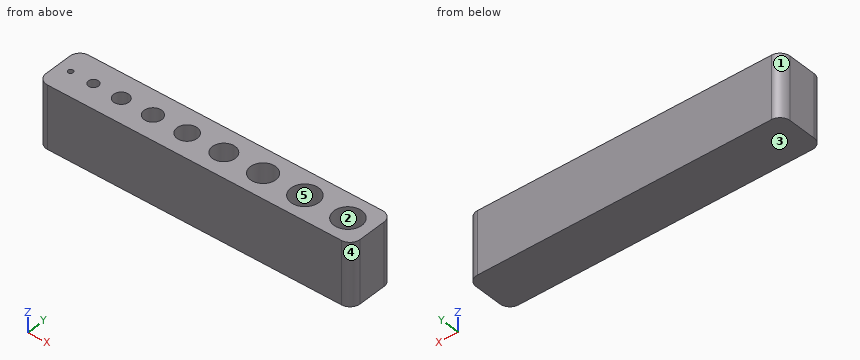
```python
from build123d import *

# Parameters (mm, degrees)
F0_W          = 62
F0_H          = 9.5
F0_R          = 0.5
F0_R_2        = 1
F0_R_3        = 1.5
F0_R_4        = 1.75
F0_R_5        = 2
F0_R_6        = 2.25
F0_R_7        = 2.5
F0_R_8        = 2.75
F1_DEPTH      = 12
F1_DEPTH_BACK = 0.4
F2_DEPTH      = 0.4
F3_R          = 2


with BuildPart() as f1:
    # F0 (on Top) → F1 (new body, two sides)
    with BuildSketch(Plane.XY) as f1_sk:
        with Locations((-1.75, 0)):
            Rectangle(F0_W, F0_H)
        with Locations((-30.25, 0)):
            Circle(F0_R, mode=Mode.SUBTRACT)
        with Locations((-25.75, 0)):
            Circle(F0_R_2, mode=Mode.SUBTRACT)
        with Locations((-20.25, 0)):
            Circle(F0_R_3, mode=Mode.SUBTRACT)
        with Locations((-14, 0)):
            Circle(F0_R_4, mode=Mode.SUBTRACT)
        with Locations((-7.25, 0)):
            Circle(F0_R_5, mode=Mode.SUBTRACT)
        Circle(F0_R_6, mode=Mode.SUBTRACT)
        with Locations((7.75, 0)):
            Circle(F0_R_7, mode=Mode.SUBTRACT)
        with Locations((16, 0)):
            Circle(F0_R_8, mode=Mode.SUBTRACT)
        with Locations((24.5, 0)):
            Circle(F0_R_8, mode=Mode.SUBTRACT)
    extrude(amount=F1_DEPTH)
    extrude(f1_sk.sketch, amount=-F1_DEPTH_BACK)

    # F0 (on Top) → F2 (join)
    with BuildSketch(Plane.XY):
        with Locations((-25.75, 0)):
            Circle(F0_R_2)
        with Locations((-20.25, 0)):
            Circle(F0_R_3)
        with Locations((-30.25, 0)):
            Circle(F0_R)
        with Locations((-14, 0)):
            Circle(F0_R_4)
        with Locations((-7.25, 0)):
            Circle(F0_R_5)
        Circle(F0_R_6)
        with Locations((7.75, 0)):
            Circle(F0_R_7)
        with Locations((16, 0)):
            Circle(F0_R_8)
        with Locations((24.5, 0)):
            Circle(F0_R_8)
    extrude(amount=-F2_DEPTH)

    # F3
    f3_edges = [f1.edges().sort_by_distance(p)[0] for p in [
        (-32.75, -4.75, 5.8),
        (29.25, -4.75, 5.8),
        (29.25, 4.75, 5.8),
        (-32.75, 4.75, 5.8),
    ]]
    fillet(f3_edges, radius=F3_R)


solid = f1.part
```
Source: CAD feature listing. Evaluate the final solid. Frame: model axes, mm. Face numbers are marked on the shaded views. A direction names the side the tool comes from. Give positions to 0.01 mm unless a question says otherwise; leave off trailing zeros. Loops run counter-clockwise (first coordinate to the right, second up) from the corner with the lowest first, then second, coordinate; pieces in that order, holes last. Notation, with made-up numbers: M 66,87 L 122,87 A5 ccw 122,91 Z; hole C -31.5,37 d10. An arc over 180 degrees is marked long. Put each result on its own line as item: value.
Q1. Section A-A (x = 0). Return the cut outline in (y, z).
Response values:
outline: M -4.75,-0.4 L 4.75,-0.4 L 4.75,12 L 2.25,12 L 2.25,0 L -2.25,0 L -2.25,12 L -4.75,12 Z
Q2. Mould query, pull axis Y, two halves, no side actions, for the marked faces 1, 2 and 3. Classes: released by +Y, released by -Y, zero draft, split by the parting line, or undercut.
Response values:
face 1: released by +Y
face 2: undercut
face 3: zero draft
Q3. Pin query (flat end, axial travel): P1, Ø2, axis at x = -8, y = 0.5, coming from the +Z side; P2, Ø1, axis at x = -26, y = -0.5, coming from the +Z side. Return the tip coordinate at first contact, or that it passes through.
Response values:
P1: stops at z = 0
P2: stops at z = 12
Q4. Reachability of the marked faces 4 and 5 from +Z, -Z, +X, -X, +Y, -Y: full face, straight path, thin tool, end or side. Return the list, or none.
Response values:
face 4: +Z, -Z, +X, -Y
face 5: +Z
Q5. Section B-B (z = 7.5). Count the separate pieces of the cut face and the enclosed holes in it, and give its area (3 significant figures).
Response values:
separate pieces: 1
enclosed holes: 9
area: 469 mm²
Q6. Line query: probe 1 along Y at (x, z) = (0, 3.5); probe 2 along Y at (x, z) = (-25.75, 6.5); probe 3 along Z at (x, y) = (6, -0.75). Output: solid intervals per line, ascending. Write a range as [from, to].
Response values:
probe 1: y = [-4.75, -2.25], [2.25, 4.75]
probe 2: y = [-4.75, -1], [1, 4.75]
probe 3: z = [-0.4, 0]
Q7. Section C-C (x = -7.25). Return the cut outline in (y, z), and give its area (3 significant figures).
Response values:
outline: M -4.75,-0.4 L 4.75,-0.4 L 4.75,12 L 2,12 L 2,0 L -2,0 L -2,12 L -4.75,12 Z
area: 69.8 mm²
